```python
from build123d import *

# Parameters (mm, degrees)
SKETCH_W       = 50
SKETCH_H       = 5
PAD_DEPTH      = 0.5
SKETCH001_W    = 45
SKETCH001_H    = 2
PAD001_DEPTH   = 5
SKETCH002_W    = 3
SKETCH002_H    = 3
SKETCH002_W_2  = 2
SKETCH002_W_3  = 1
SKETCH002_W_4  = 0.9
SKETCH002_W_5  = 0.8
SKETCH002_W_6  = 0.7
SKETCH002_W_7  = 0.6
SKETCH002_W_8  = 0.5
SKETCH002_W_9  = 0.4
SKETCH002_W_10 = 0.2
SKETCH002_W_11 = 0.1
POCKET_DEPTH   = 3.501


with BuildPart() as part:
    # Sketch → Pad (new body)
    with BuildSketch(Plane.XY):
        Rectangle(SKETCH_W, SKETCH_H)
    extrude(amount=PAD_DEPTH)

    # Sketch001 (on Face6 of Pad) → Pad001 (join)
    with BuildSketch(Plane.XY.offset(0.5)):
        Rectangle(SKETCH001_W, SKETCH001_H)
    extrude(amount=PAD001_DEPTH)

    # Sketch002 (on Face7 of Pad001) → Pocket (cut, through all)
    with BuildSketch(Plane.XZ.offset(1)):
        with Locations((19, 3)):
            Rectangle(SKETCH002_W, SKETCH002_H)
        with Locations((13.5, 3)):
            Rectangle(SKETCH002_W_2, SKETCH002_H)
        with Locations((9, 3)):
            Rectangle(SKETCH002_W_3, SKETCH002_H)
        with Locations((5.05, 3)):
            Rectangle(SKETCH002_W_4, SKETCH002_H)
        with Locations((1.2, 3)):
            Rectangle(SKETCH002_W_5, SKETCH002_H)
        with Locations((-2.55, 3)):
            Rectangle(SKETCH002_W_6, SKETCH002_H)
        with Locations((-6.2, 3)):
            Rectangle(SKETCH002_W_7, SKETCH002_H)
        with Locations((-9.75, 3)):
            Rectangle(SKETCH002_W_8, SKETCH002_H)
        with Locations((-13.2, 3)):
            Rectangle(SKETCH002_W_9, SKETCH002_H)
        with Locations((-16.5, 3)):
            Rectangle(SKETCH002_W_10, SKETCH002_H)
        with Locations((-19.65, 3)):
            Rectangle(SKETCH002_W_11, SKETCH002_H)
    extrude(amount=-POCKET_DEPTH, mode=Mode.SUBTRACT)


solid = part.part
```
Design review of the part built by this model. Coordinates are the model's own, in mm. A direction names the side the tool comes from. Round coordinates to 2 decimals unless told otherwise and drop trailing zeros. Order: outer loops, then holes, each group sorted by start corner. A loop starts at its lowest first (then second) coordinate and runs counter-clockwise, first axis right, second up. Notation, with made-up numbers: M 82,-10 L 99,-10 A15 ccw 99,1 Z; hole C -16.75,10 d2. An arc over 180 degrees is marked long. Put each result on its own line as item: value.
Q1. Consider section A-A (x = -14.5). State the section outline as (y, z) points, and give its area (3 significant figures).
Reported:
outline: M -2.5,0 L 2.5,0 L 2.5,0.5 L 1,0.5 L 1,5.5 L -1,5.5 L -1,0.5 L -2.5,0.5 Z
area: 12.5 mm²
Q2. To check wall thickness, follow line 1 (X direction, y = -0.9, z = 4.8); line 2 (Y direction, x = 12, z = 1.55); line 3 (Z direction, x = -16.5, y = 0.45). State the ranges of each line that lie inside material, in increasing order.
Reported:
line 1: -22.5 to 22.5
line 2: -1 to 1
line 3: 0 to 1.5, 4.5 to 5.5
Q3. Draft analysis for pull direction X (two halves, no side actions). For faces 1 (the face through (-13, 0, 3)), 2 (the face through (0, 2, 0.5)), 3 (the face through (22.5, 0, 3)), state which applies: released by +X, released by -X, zero draft, split by the parting line, or undercut.
Reported:
face 1: undercut
face 2: zero draft
face 3: released by +X
Q4. Machinability: for faces 4 (the face through (-22.5, 0, 3)), 5 (the face through (5.5, 0, 3)), 6 (the face through (0, 0, 5.5)), which of the approach directions +Z, -Z, +X, -X, +Y, -Y give a long, thin tool a straight path to every point of the face, cutting with its end or side? Answer none if there is none.
Reported:
face 4: +Z, -X, +Y, -Y
face 5: +Y, -Y
face 6: +Z, +X, -X, +Y, -Y
Q5. Consider section C-C (y = 1.85). State the section outline as (x, z) points, and give its area (3 significant figures).
Reported:
outline: M -25,0 L 25,0 L 25,0.5 L -25,0.5 Z
area: 25.0 mm²
Q6. Insertion check: pin 1 Ø1.6 at (y, z) = (0.5, 2.5) entering from -X; pin 2 Ø1.5 at (x, z) = (-7, 3.5) entering from +Y; pin 3 Ø2 at (y, z) = (0, 3) entering from +X. Each pin has a flat end and moves straight along its axis. Give the tip position at first contact, or say it passes through.
Reported:
pin 1: x = -22.5
pin 2: y = 1
pin 3: x = 22.5
Q7. Consider section B-B (z = 4). State how many separate pieces and enclosed holes the cut face has, and give its area (3 significant figures).
Reported:
separate pieces: 12
enclosed holes: 0
area: 69.6 mm²
